```python
from build123d import *

# Parameters (mm, degrees)
SKETCH1_W                      = 19.5
SKETCH1_H                      = 16
EXTRUDE1_DEPTH                 = 7.95
CBORE_FOR_M6_SHCS1_D           = 6.6
CBORE_FOR_M6_SHCS1_CBORE_D     = 11
CBORE_FOR_M6_SHCS1_CBORE_DEPTH = 6
CHAMFER1_SIZE                  = 0.762
CHAMFER2_SIZE                  = 1.5748


with BuildPart() as part:
    # Sketch1 → Extrude1 (new, symmetric)
    with BuildSketch(Plane(origin=(0, 0, 0), x_dir=(1, 0, 0), z_dir=(0, 1, 0))):
        Rectangle(SKETCH1_W, SKETCH1_H)
    extrude(amount=EXTRUDE1_DEPTH, both=True)

    # CBORE for M6 SHCS1 (through all)
    with Locations(Plane.XY.offset(8)):
        with Locations((0, 0)):
            CounterBoreHole(CBORE_FOR_M6_SHCS1_D / 2, CBORE_FOR_M6_SHCS1_CBORE_D / 2, CBORE_FOR_M6_SHCS1_CBORE_DEPTH)

    # Chamfer1
    chamfer1_edges = [part.edges().sort_by_distance(p)[0] for p in [
        (9.75, 7.95, 0),
        (0, 7.95, -8),
        (-9.75, 7.95, 0),
        (0, -7.95, -8),
        (9.75, -7.95, 0),
        (-9.75, -7.95, 0),
        (-9.75, 0, -8),
        (9.75, 0, -8),
    ]]
    chamfer(chamfer1_edges, length=CHAMFER1_SIZE)

    # Chamfer2
    chamfer2_edges = [part.edges().sort_by_distance(p)[0] for p in [
        (0, -7.95, 8),
        (0, 7.95, 8),
    ]]
    chamfer(chamfer2_edges, length=CHAMFER2_SIZE)


solid = part.part
```
Geometry check sheet. Reference: the model listing, model coordinates, mm. A direction names the side the tool comes from. Coordinates: 2 decimals unless noted, no trailing zeros. Order: outer loops, then holes, each group sorted by start corner. A loop starts at its lowest first (then second) coordinate and runs counter-clockwise, first axis right, second up. Notation, with made-up numbers: (25.25, 49) - (59.25, 49) arc R16 cw to (59.25, 66) - close; hole circle Ø10 at (87.25, 28). An arc over 180 degrees is marked (long way). Answer in a Markdown table with one row per item. Add a question column.
1. Section check B-B (z = 1.75). Enter the section's corners in (x, y), plus the area to 3 significant figures.
2. Access from +Z, -Z, +X, -X, +Y, -Y to the whole of each face (thin tool, end or side, straight path). Record for faces 5 (the face through (-2, 3, -8)), 6 (the face through (-1.19, -5.37, 5.04)).
3. Section check C-C (y = 0). Enter the section's corners in (x, z), plus the area to 3 significant figures.
4. Section check D-D (x = -4.75). Enter the section's corners in (y, z), plus the area to 3 significant figures.
5. Draft check along X on faces 1 (the face through (-9.75, 0, 0)), 2 (the face through (9.75, 0, 0)), 3 (the face through (0, -6, 8)), 4 (the face through (4, 0, 2)). Enter one of: +X half, -X half, draft (parallel to the pull), parting line (faces both ways), or undercut.
6. Section check A-A (x = 0). Enter the section's corners in (y, z), plus the area to 3 significant figures.
7. Gauge pin test, flat end, axial feed: pin 1 Ø8.5 at (x, y) = (0, 0) entering from +Z. Record the tip position at first contact, or that the pin passes through.
8. Material ranges on L1, parallel to Y at x = 0, z = 6; L2, parallel to Y at x = 0, z = -1.25; L3, parallel to X at y = -1, z = -6.25, recorded low to high. Write a range as [from, to].
Data:
| question | item | result |
|---|---|---|
| 1 | outline | (-9.75, -7.19) - (-8.99, -7.95) - (8.99, -7.95) - (9.75, -7.19) - (9.75, 7.19) - (8.99, 7.95) - (-8.99, 7.95) - (-9.75, 7.19) - close; hole circle Ø6.6 at (0, 0) |
| 1 | area | 275 mm² |
| 2 | face 5 | -Z, +X, -X, +Y, -Y |
| 2 | face 6 | +Z |
| 3 | outline | (-9.75, -7.24) - (-8.99, -8) - (-3.3, -8) - (-3.3, 2) - (-5.5, 2) - (-5.5, 8) - (-9.75, 8) - close; (3.3, -8) - (8.99, -8) - (9.75, -7.24) - (9.75, 8) - (5.5, 8) - (5.5, 2) - (3.3, 2) - close |
| 3 | area | 179 mm² |
| 4 | outline | (-7.95, -7.24) - (-7.19, -8) - (7.19, -8) - (7.95, -7.24) - (7.95, 6.43) - (6.38, 8) - (2.77, 8) - (2.77, 2) - (-2.77, 2) - (-2.77, 8) - (-6.38, 8) - (-7.95, 6.43) - close |
| 4 | area | 218 mm² |
| 5 | face 1 | -X half |
| 5 | face 2 | +X half |
| 5 | face 3 | draft |
| 5 | face 4 | undercut |
| 6 | outline | (-7.95, -7.24) - (-7.19, -8) - (-3.3, -8) - (-3.3, 2) - (-5.5, 2) - (-5.5, 8) - (-6.38, 8) - (-7.95, 6.43) - close; (3.3, -8) - (7.19, -8) - (7.95, -7.24) - (7.95, 6.43) - (6.38, 8) - (5.5, 8) - (5.5, 2) - (3.3, 2) - close |
| 6 | area | 119 mm² |
| 7 | pin 1 | stops at z = 2 |
| 8 | L1 | y = [-7.95, -5.5], [5.5, 7.95] |
| 8 | L2 | y = [-7.95, -3.3], [3.3, 7.95] |
| 8 | L3 | x = [-9.75, -3.14], [3.14, 9.75] |
